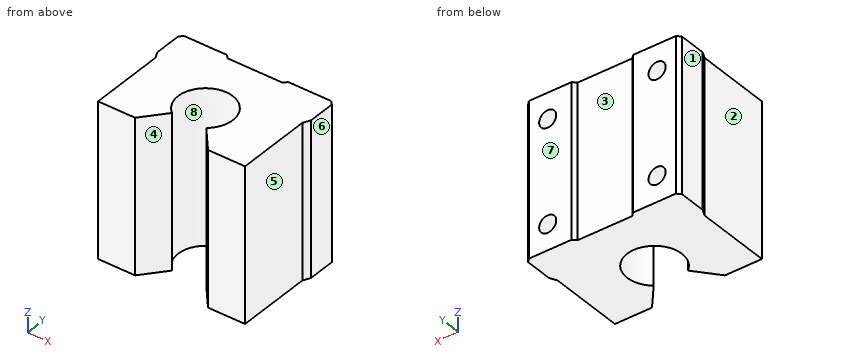
```python
from build123d import *

# Parameters (mm, degrees)
DODANIE_WYCI_GNI_CIE1_DEPTH = 45
SZKIC2_R                    = 2.5
WYTNIJ_WYCI_GNI_CIE1_DEPTH  = 12


with BuildPart() as part:
    # Szkic1 → Dodanie-wyciągnięcie1 (new body)
    with BuildSketch(Plane.XY):
        with BuildLine():
            Line((8, 32), (-8, 32))
            Line((-8, 32), (-9, 33))
            Line((-9, 33), (-21.5, 33))
            Line((-21.5, 33), (-22.5, 32))
            Line((-22.5, 32), (-22.5, 24))
            Line((-22.5, 24), (-21.5, 22))
            Line((-21.5, 22), (-21.5, 0))
            Line((-21.5, 0), (-10.668119688, 0))
            Line((-10.668119688, 0), (-5, 6.755002002))
            ThreePointArc((-5, 6.755002002), (0, 21), (5, 6.755002002))
            Line((5, 6.755002002), (10.668119688, 0))
            Line((10.668119688, 0), (21.5, 0))
            Line((21.5, 0), (21.5, 22))
            Line((21.5, 22), (22.5, 24))
            Line((22.5, 24), (22.5, 32))
            Line((22.5, 32), (21.5, 33))
            Line((21.5, 33), (9, 33))
            Line((9, 33), (8, 32))
        make_face()
    extrude(amount=DODANIE_WYCI_GNI_CIE1_DEPTH)

    # Szkic2 → Wytnij-wyciągnięcie1 (cut)
    with BuildSketch(Plane(origin=(0, 33, 0), x_dir=(1, 0, 0), z_dir=(0, 1, 0))):
        with Locations(Location((-16, -37.5, 0), (0, 0, 270))):
            Circle(SZKIC2_R)
        with Locations(Location((-16, -7.5, 0), (0, 0, 270))):
            Circle(SZKIC2_R)
        with Locations(Location((16, -7.5, 0), (0, 0, 270))):
            Circle(SZKIC2_R)
        with Locations(Location((16, -37.5, 0), (0, 0, 270))):
            Circle(SZKIC2_R)
    extrude(amount=-WYTNIJ_WYCI_GNI_CIE1_DEPTH, mode=Mode.SUBTRACT)

    # Wytnij-wyciągnięcie2 cone 1 section (through the dimple's axis) → Wytnij-wyciągnięcie2 (revolve, cut)
    with BuildSketch(Plane(origin=(16, 21, 7.5), x_dir=(0, 0, 1), z_dir=(1, 0, 0))):
        Polygon((0, 0), (2.5, 0), (0, 1.56217338), align=None)
    revolve(axis=Axis((16, 21, 7.5), (0, -1, 0)), mode=Mode.SUBTRACT)

    # Wytnij-wyciągnięcie2 cone 2 section (through the dimple's axis) → Wytnij-wyciągnięcie2 cone 2 (revolve, cut)
    with BuildSketch(Plane(origin=(-16, 21, 7.5), x_dir=(0, 0, 1), z_dir=(1, 0, 0))):
        Polygon((0, 0), (2.5, 0), (0, 1.56217338), align=None)
    revolve(axis=Axis((-16, 21, 7.5), (0, -1, 0)), mode=Mode.SUBTRACT)

    # Wytnij-wyciągnięcie2 cone 3 section (through the dimple's axis) → Wytnij-wyciągnięcie2 cone 3 (revolve, cut)
    with BuildSketch(Plane(origin=(-16, 21, 37.5), x_dir=(0, 0, 1), z_dir=(1, 0, 0))):
        Polygon((0, 0), (2.5, 0), (0, 1.56217338), align=None)
    revolve(axis=Axis((-16, 21, 37.5), (0, -1, 0)), mode=Mode.SUBTRACT)

    # Wytnij-wyciągnięcie2 cone 4 section (through the dimple's axis) → Wytnij-wyciągnięcie2 cone 4 (revolve, cut)
    with BuildSketch(Plane(origin=(16, 21, 37.5), x_dir=(0, 0, 1), z_dir=(1, 0, 0))):
        Polygon((0, 0), (2.5, 0), (0, 1.56217338), align=None)
    revolve(axis=Axis((16, 21, 37.5), (0, -1, 0)), mode=Mode.SUBTRACT)


solid = part.part
```
Read the model definition and answer for the solid it produces. Units are mm, in the model's axes. Face numbers are marked on the shaded views. A direction names the side the tool comes from. Give positions to 0.01 mm unless a question says otherwise; leave off trailing zeros. Loops run counter-clockwise (first coordinate to the right, second up) from the corner with the lowest first, then second, coordinate; pieces in that order, holes last.
Item 1: The part is cut by section A-A (y = 13). Write down the section's boundary in (x, z), and give its area (4 significant figures).
Item 2: The part is cut by section B-B (x = 6.5). Write down the section's boundary in (y, z).
Item 3: The part is cut by section C-C (z = 18). Write down the section's boundary in (x, y) (3 decimals).
Item 4: The part is cut by section D-D (x = 0). Write down the section's boundary in (y, z).
Item 5: The mould has two halves that part along X. Classify the marked faces 6, 7 and 8: released by +X, released by -X, zero draft, split by the parting line, or undercut.
Item 6: Find the intervals of material crossed by line 1 along X through (y, z) = (28, 37.5); line 2 along X through (y, z) = (24, 7); line 3 along Y through (x, z) = (-6, 41.5), in increasing order.
Item 7: For the marked faces 1, 2, 3, 4 and 5, determine the directions among +Z, -Z, +X, -X, +Y, -Y from which every point of the face is accessible in a straight line to the end or side of a thin tool.
Item 8: Each of these flat-tipped pins is pushed along its axis until it touches: pin 1 Ø12 at (y, z) = (5, 30.5) entering from -X; pin 2 Ø4 at (x, z) = (-16, 37.5) entering from +Y; pin 3 Ø4 at (y, z) = (11, 28) entering from +X; pin 4 Ø9.5 at (x, y) = (0, 13) entering from -Z. Where does it stop, or does it pass through?
Taken from the geometry:
1. outline: (-21.5, 0) - (-8, 0) - (-8, 45) - (-21.5, 45) - close; (8, 0) - (21.5, 0) - (21.5, 45) - (8, 45) - close
1. area: 1,215 mm2
2. outline: (4.97, 0) - (8.34, 0) - (8.34, 45) - (4.97, 45) - close; (17.66, 0) - (32, 0) - (32, 45) - (17.66, 45) - close
3. outline: (-22.5, 24) - (-21.5, 22) - (-21.5, 0) - (-10.668, 0) - (-5, 6.755) arc R8 cw (long way) to (5, 6.755) - (10.668, 0) - (21.5, 0) - (21.5, 22) - (22.5, 24) - (22.5, 32) - (21.5, 33) - (9, 33) - (8, 32) - (-8, 32) - (-9, 33) - (-21.5, 33) - (-22.5, 32) - close
4. outline: (21, 0) - (32, 0) - (32, 45) - (21, 45) - close
5. face 6: released by +X
5. face 7: zero draft
5. face 8: undercut
6. line 1: x = -22.5 to -18.5, -13.5 to 13.5, 18.5 to 22.5
6. line 2: x = -22.5 to -18.45, -13.55 to 13.55, 18.45 to 22.5
6. line 3: y = 5.56 to 7.71, 18.29 to 32
7. face 1: +Z, -Z, -X, +Y, -Y
7. face 2: +Z, -Z, -X, -Y
7. face 3: +Z, -Z, +Y
7. face 4: +Z, -Z, -Y
7. face 5: +Z, -Z, +X, -Y
8. pin 1: stops at x = -21.5
8. pin 2: stops at y = 20.69
8. pin 3: stops at x = 21.5
8. pin 4: passes through
